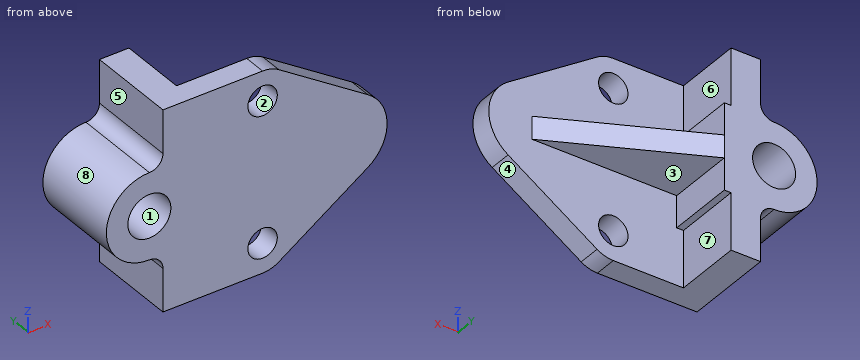
from build123d import *

# Parameters (mm, degrees)
BOSS_EXTRUDE1_DEPTH      = 20
BOSS_EXTRUDE1_DEPTH_BACK = 20
CUT_EXTRUDE1_START       = -30
CUT_EXTRUDE1_DEPTH       = 30
BOSS_EXTRUDE2_START      = -44
BOSS_EXTRUDE2_DEPTH      = 5
HOLE1_D                  = 19
HOLE2_D                  = 13


with BuildPart() as part:
    # Sketch1 → Boss-Extrude1 (new, two sides: drawn at the far end of the back side and taken through both)
    with BuildSketch(Plane(origin=(0, 0, 0), x_dir=(1, 0, 0), z_dir=(0, 1, 0)).offset(-BOSS_EXTRUDE1_DEPTH_BACK)):
        with BuildLine():
            Line((6, 25), (6, 44))
            Line((6, 44), (50, 44))
            ThreePointArc((50, 44), (53.744006319, 43.449193415), (57.170747509, 41.843448721))
            Line((57.170747509, 41.843448721), (96.480323283, 15.848117361))
            ThreePointArc((96.480323283, 15.848117361), (105, 0), (96.480323283, -15.848117361))
            Line((96.480323283, -15.848117361), (57.170747509, -41.843448721))
            ThreePointArc((57.170747509, -41.843448721), (53.744006319, -43.449193415), (50, -44))
            Line((50, -44), (6, -44))
            Line((6, -44), (6, -25))
            ThreePointArc((6, -25), (4.242640687, -20.757359313), (0, -19))
            ThreePointArc((0, -19), (-19, 0), (0, 19))
            ThreePointArc((0, 19), (4.242640687, 20.757359313), (6, 25))
        make_face()
    extrude(amount=BOSS_EXTRUDE1_DEPTH + BOSS_EXTRUDE1_DEPTH_BACK)

    # Sketch2 → Cut-Extrude1 (cut)
    with BuildSketch(Plane(origin=(0, 20, 0), x_dir=(1, 0, 0), z_dir=(0, 1, 0)).offset(CUT_EXTRUDE1_START)):
        with BuildLine():
            Line((19, 44), (19, 19))
            Line((19, 19), (22, 19))
            Line((22, 19), (22, -19))
            Line((22, -19), (19, -19))
            Line((19, -19), (19, -44))
            Line((19, -44), (50, -44))
            ThreePointArc((50, -44), (53.744006319, -43.449193415), (57.170747509, -41.843448721))
            Line((57.170747509, -41.843448721), (96.480323283, -15.848117361))
            ThreePointArc((96.480323283, -15.848117361), (105, 0), (96.480323283, 15.848117361))
            Line((96.480323283, 15.848117361), (57.170747509, 41.843448721))
            ThreePointArc((57.170747509, 41.843448721), (53.744006319, 43.449193415), (50, 44))
            Line((50, 44), (19, 44))
        make_face()
    extrude(amount=CUT_EXTRUDE1_DEPTH, mode=Mode.SUBTRACT)

    # Sketch3 → Boss-Extrude2 (add, symmetric)
    with BuildSketch(Plane.XY.offset(44).offset(BOSS_EXTRUDE2_START)):
        Polygon((22, 20), (86, -10), (57.170747509, -10), (50, -10), (22, -10), align=None)
    extrude(amount=BOSS_EXTRUDE2_DEPTH, both=True)

    # Hole1 (through all)
    with Locations(Plane(origin=(0, 20, 0), x_dir=(1, 0, 0), z_dir=(0, 1, 0))):
        with Locations((0, 0)):
            Hole(HOLE1_D / 2)

    # Hole2 (through all)
    with Locations(Plane(origin=(0, -10, 0), x_dir=(1, 0, 0), z_dir=(0, 1, 0))):
        with Locations((50, -31), (50, 31)):
            Hole(HOLE2_D / 2)


solid = part.part
Check sheet for the modelled part. Datum: model origin and axes. Units: mm. Face numbers are marked on the shaded views. A direction names the side the tool comes from. Round coordinates to 2 decimals unless told otherwise and drop trailing zeros. Loops run counter-clockwise (first coordinate to the right, second up) from the corner with the lowest first, then second, coordinate; pieces in that order, holes last. Notation, with made-up numbers: M 84,20 L 92,20 A17 cw 92,28 Z; hole C -32.5,27 d1. An arc over 180 degrees is marked long. One line per item, written item: value.
(1) Sectioned sample at C-C, the plane y = -14. Record the cut outline in (x, z), then the cut area to 3 significant figures.
Computed values:
outline: M 0,-19 A6 cw 6,-25 L 6,-44 L 50,-44 A13 ccw 57.17,-41.84 L 96.48,-15.85 A19 ccw 96.48,15.85 L 57.17,41.84 A13 ccw 50,44 L 6,44 L 6,25 A6 cw 0,19 A19 ccw Z; hole C 0,0 d19; hole C 50,-31 d13; hole C 50,31 d13
area: 7,210 mm^2
(2) Thickness scan on line 1 (Z direction, x = 50, y = -14); line 2 (X direction, y = -12.25, z = -31); line 3 (Y direction, x = 84.5, z = 8.5). Record the ranges inside material, lowest first.
Computed values:
line 1: z = -44 to -37.5, -24.5 to 24.5, 37.5 to 44
line 2: x = 6 to 43.5, 56.5 to 73.57
line 3: y = -20 to -10
(3) Depth check by flat-ended pin: pin 1 Ø3 at (x, z) = (48.5, 7.5) entering from +Y; pin 2 Ø9.5 at (y, z) = (4.5, 38) entering from -X; pin 3 Ø12.5 at (y, z) = (12.5, 29) entering from +X. Enter the tip coordinate at first touch or a pass-through.
Computed values:
pin 1: stops at y = -10
pin 2: stops at x = 6
pin 3: stops at x = 19
(4) Sectioned sample at D-D, the plane x = 46. Record the cut outline in (y, z).
Computed values:
outline: M -20,-44 L -10,-44 L -10,-36.12 L -20,-36.12 Z; M -20,-25.88 L -10,-25.88 L -10,-5 L 8.75,-5 L 8.75,5 L -10,5 L -10,25.88 L -20,25.88 Z; M -20,36.12 L -10,36.12 L -10,44 L -20,44 Z
(5) Access from +Z, -Z, +X, -X, +Y, -Y to the whole of each face (thin tool, end or side, straight path). Record for the marked faces 5, 6, 7 and 8.
Computed values:
face 5: +Z, -X, +Y, -Y
face 6: +Z, +X, +Y
face 7: -Z, +X, +Y
face 8: -X, +Y, -Y
(6) Release check for a two-part mould opening along X. For the marked faces 1, 2, 3 and 4 record: +X half, -X half, draft (parallel to the pull), parting line (faces both ways), or undercut.
Computed values:
face 1: undercut
face 2: undercut
face 3: draft
face 4: +X half
(7) Sectioned sample at B-B, the plane z = 0. Record the cut outline in (x, y), then the cut area to 3 significant figures.
Computed values:
outline: M -19,-20 L -9.5,-20 L -9.5,20 L -19,20 Z; M 9.5,-20 L 105,-20 L 105,-10 L 86,-10 L 22,20 L 9.5,20 Z
area: 2,670 mm^2
(8) Sectioned sample at A-A, the plane y = 14. Record the cut outline in (x, z).
Computed values:
outline: M 0,-19 A6 cw 6,-25 L 6,-44 L 19,-44 L 19,-19 L 22,-19 L 22,-5 L 34.8,-5 L 34.8,5 L 22,5 L 22,19 L 19,19 L 19,44 L 6,44 L 6,25 A6 cw 0,19 A19 ccw Z; hole C 0,0 d19
